from build123d import *

# Parameters (mm, degrees)
BOSS_EXTRUDE1_DEPTH = 3
CUT_EXTRUDE1_DEPTH  = 10


with BuildPart() as part:
    # Sketch1 → Boss-Extrude1 (new body)
    with BuildSketch(Plane(origin=(0, 0, 0), x_dir=(1, 0, 0), z_dir=(0, 1, 0))):
        Polygon((-72.98636562, 0), (72.98636562, 0), (74.075, 77), (-74.075, 77), align=None)
    extrude(amount=BOSS_EXTRUDE1_DEPTH)

    # Sketch2 → Cut-Extrude1 (cut)
    with BuildSketch(Plane(origin=(0, 3, 0), x_dir=(1, 0, 0), z_dir=(0, 1, 0))):
        with BuildLine():
            Line((-46.75, 67), (-53.932619531, 67))
            ThreePointArc((-53.932619531, 67), (-61.003687343, 64.071067812), (-63.932619531, 57))
            Line((-63.932619531, 57), (-63.932619531, 20))
            ThreePointArc((-63.932619531, 20), (-61.003687343, 12.928932188), (-53.932619531, 10))
            Line((-53.932619531, 10), (-46.75, 10))
            ThreePointArc((-46.75, 10), (-39.678932188, 12.928932188), (-36.75, 20))
            Line((-36.75, 20), (-36.75, 57))
            ThreePointArc((-36.75, 57), (-39.678932188, 64.071067812), (-46.75, 67))
        make_face()
        with BuildLine():
            Line((-13.25, 67), (0, 67))
            Line((0, 67), (0, 10))
            Line((0, 10), (-13.25, 10))
            ThreePointArc((-13.25, 10), (-20.321067812, 12.928932188), (-23.25, 20))
            Line((-23.25, 20), (-23.25, 57))
            ThreePointArc((-23.25, 57), (-20.321067812, 64.071067812), (-13.25, 67))
        make_face()
    cut_extrude1 = extrude(amount=-CUT_EXTRUDE1_DEPTH, mode=Mode.SUBTRACT)

    # Mirror1: Cut-Extrude1 across plane
    add(cut_extrude1.mirror(Plane(origin=(0, 0, 0), x_dir=(0, 0, 1), z_dir=(1, 0, 0))), mode=Mode.SUBTRACT)


solid = part.part
Here's how the part is built. I have some questions about the finished solid (model axes, mm). Round coordinates to 2 decimals unless told otherwise and drop trailing zeros. Order: outer loops, then holes, each group sorted by start corner. A loop starts at its lowest first (then second) coordinate and runs counter-clockwise, first axis right, second up. Notation, with made-up numbers: M 72.25,24.25 L 124.25,24.25 A35 cw 124.25,62.25 Z; hole C -32,38.25 d2. An arc over 180 degrees is marked long. Return JSON: item names as keys, results as strings. Group by question number.
1. If we section it at A-A on x = 5: List the corners of the cut face in (y, z) for me.
2. If we mould it in two halves opening along Z, with no side actions, what happens to faces 1 (the face through (60.926, 1.521, -64.148)), 2 (the face through (1, 1, -77)), 3 (the face through (-1, 1, 0))? For each: pulls with the +Z half, pulls with the -Z half, needs draft (parallel to the pull), parting line crosses it, or undercut.
3. Please list where these lines run through material, in increasing order: probe 1 along X at (y, z) = (1.1, -18); probe 2 along X at (y, z) = (0.7, -51); probe 3 along Z at (x, y) = (-13, 0.7).
4. If we section it at C-C on z = -13: List the corners of the cut face in (x, y) for me.
5. I'm going to push flat-ended pins straight in: pin 1 Ø8 at (x, z) = (-34, -64.5) entering from -Y; pin 2 Ø1.5 at (y, z) = (2, -46.5) entering from -X; pin 3 Ø1.5 at (y, z) = (2, -45) entering from +X. Where does each tip first touch, or does it pass through?
6. If we section it at B-B on y = 0.65: List the corners of the cut face in (x, z) for me (3 decimals), then the cut area to 3 significant figures.
7. If we section it at D-D on z = -33: List the corners of the cut face in (x, y) for me, then the cut area to 3 significant figures.
Reply:
{
 "1": {"outline": "M 0,-77 L 3,-77 L 3,-67 L 0,-67 Z; M 0,-10 L 3,-10 L 3,0 L 0,0 Z"},
 "2": {"face 1": "undercut", "face 2": "pulls with the -Z half", "face 3": "pulls with the +Z half"},
 "3": {"probe 1": "-73.24 to -63.73, -36.95 to -23.05, 23.05 to 36.95, 63.73 to 73.24", "probe 2": "-73.71 to -63.93, -36.75 to -23.25, 23.25 to 36.75, 63.93 to 73.71", "probe 3": "-77 to -67, -10 to 0"},
 "4": {"outline": "M -73.17,0 L -61.07,0 L -61.07,3 L -73.17,3 Z; M -39.61,0 L -20.39,0 L -20.39,3 L -39.61,3 Z; M 20.39,0 L 39.61,0 L 39.61,3 L 20.39,3 Z; M 61.07,0 L 73.17,0 L 73.17,3 L 61.07,3 Z"},
 "5": {"pin 1": "y = 0", "pin 2": "x = -73.65", "pin 3": "x = 73.63"},
 "6": {"outline": "M -74.075,-77 L 74.075,-77 L 72.986,0 L -72.986,0 Z; hole M -63.933,-57 A10 ccw -53.933,-67 L -46.75,-67 A10 ccw -36.75,-57 L -36.75,-20 A10 ccw -46.75,-10 L -53.933,-10 A10 ccw -63.933,-20 Z; hole M -23.25,-57 A10 ccw -13.25,-67 L 13.25,-67 A10 ccw 23.25,-57 L 23.25,-20 A10 ccw 13.25,-10 L -13.25,-10 A10 ccw -23.25,-20 Z; hole M 36.75,-57 A10 ccw 46.75,-67 L 53.933,-67 A10 ccw 63.933,-57 L 63.933,-20 A10 ccw 53.933,-10 L 46.75,-10 A10 ccw 36.75,-20 Z", "area": "5,830 mm^2"},
 "7": {"outline": "M -73.45,0 L -63.93,0 L -63.93,3 L -73.45,3 Z; M -36.75,0 L -23.25,0 L -23.25,3 L -36.75,3 Z; M 23.25,0 L 36.75,0 L 36.75,3 L 23.25,3 Z; M 63.93,0 L 73.45,0 L 73.45,3 L 63.93,3 Z", "area": "138 mm^2"}
}
